from build123d import *

# Parameters (mm, degrees)
SKETCH_1_R          = 235
EXTRUDE_1_DEPTH     = 5
SKETCH_2_R          = 235
SKETCH_2_R_2        = 230
EXTRUDE_2_DEPTH     = 170
CUT_EXTRUDE_1_DEPTH = 376.599520766
EXTRUDE_START       = -5
EXTRUDE_3_DEPTH     = 5
EXTRUDE_4_DEPTH     = 5
SKETCH_6_R          = 2
CUT_EXTRUDE_2_DEPTH = 5
FILLET_1_R          = 3
EXTRUDE_5_DEPTH     = 5
FILLET_2_R          = 10
FILLET_3_R          = 10
SKETCH_8_R          = 2
CUT_EXTRUDE_3_DEPTH = 5
FILLET_4_R          = 10
EXTRUDE_6_DEPTH     = 4
FILLET_5_R          = 3
EXTRUDE_7_DEPTH     = 20
CUT_EXTRUDE_START   = 120
SKETCH_12_W         = 22.896395415
SKETCH_12_H         = 51.404652451
CUT_EXTRUDE_5_DEPTH = 120
SKETCH_13_W         = 30
SKETCH_13_H         = 30
CUT_EXTRUDE_6_DEPTH = 378.955023951
FILLET_6_R          = 5
CUT_EXTRUDE_7_DEPTH = 10
SKETCH_15_R         = 1.5
CUT_EXTRUDE_8_DEPTH = 10
CHAMFER_1_SIZE      = 0.5
SKETCH_16_R         = 2
CUT_EXTRUDE_9_DEPTH = 10
CHAMFER_2_SIZE      = 0.5


with BuildPart() as part:
    # 草图1 → 凸台-拉伸1 (new body)
    with BuildSketch(Plane(origin=(0, 0, 0), x_dir=(0, 0, -1), z_dir=(1, 0, 0))):
        Circle(SKETCH_1_R)
    extrude(amount=EXTRUDE_1_DEPTH)

    # 草图2 → 凸台-拉伸2 (add)
    with BuildSketch(Plane(origin=(5, 0, 0), x_dir=(0, 0, -1), z_dir=(1, 0, 0))):
        Circle(SKETCH_2_R)
        Circle(SKETCH_2_R_2, mode=Mode.SUBTRACT)
    extrude(amount=EXTRUDE_2_DEPTH)

    # 草图3 → 切除-拉伸1 (cut, through all)
    with BuildSketch(Plane.ZY):
        Polygon((0, 0), (0, 250), (330.887429436, 250), (330.887429436, -253.432712339), (-250, -253.432712339), (-250, 0), align=None)
    extrude(amount=-CUT_EXTRUDE_1_DEPTH, mode=Mode.SUBTRACT)

    # 草图4 → 凸台-拉伸3 (add)
    with BuildSketch(Plane(origin=(167, 0, 0), x_dir=(0, 0, -1), z_dir=(1, 0, 0)).offset(EXTRUDE_START)):
        with BuildLine():
            Line((170.570968163, 130.883707237), (182.471268267, 140.015128672))
            ThreePointArc((182.471268267, 140.015128672), (162.634559673, 162.634559673), (140.015128672, 182.471268267))
            Line((140.015128672, 182.471268267), (130.883707237, 170.570968163))
            ThreePointArc((130.883707237, 170.570968163), (152.027957955, 152.027957955), (170.570968163, 130.883707237))
        make_face()
    extrude(amount=EXTRUDE_3_DEPTH)

    # 草图5 → 凸台-拉伸4 (add)
    with BuildSketch(Plane(origin=(59, 0, 0), x_dir=(0, 0, -1), z_dir=(1, 0, 0)).offset(EXTRUDE_START)):
        with BuildLine():
            Line((170.570968163, 130.883707237), (182.471268267, 140.015128672))
            ThreePointArc((182.471268267, 140.015128672), (162.634559673, 162.634559673), (140.015128672, 182.471268267))
            Line((140.015128672, 182.471268267), (130.883707237, 170.570968163))
            ThreePointArc((130.883707237, 170.570968163), (152.027957955, 152.027957955), (170.570968163, 130.883707237))
        make_face()
    extrude(amount=EXTRUDE_4_DEPTH)

    # 草图6 → 切除-拉伸2 (cut)
    with BuildSketch(Plane(origin=(167, 0, 0), x_dir=(0, 0, -1), z_dir=(1, 0, 0))):
        with Locations((146.301163465, 168.30023639)):
            Circle(SKETCH_6_R)
        with Locations((168.30023639, 146.301163465)):
            Circle(SKETCH_6_R)
    extrude(amount=-CUT_EXTRUDE_2_DEPTH, mode=Mode.SUBTRACT)

    # 圆角1
    fillet_1_edges = [part.edges().sort_by_distance(p)[0] for p in [
        (5, 162.634559673, -162.634559673),
        (0, 166.170093579, -166.170093579),
    ]]
    fillet(fillet_1_edges, radius=FILLET_1_R)

    # 草图7 → 凸台-拉伸5 (add)
    with BuildSketch(Plane(origin=(175, 0, 0), x_dir=(0, 0, -1), z_dir=(1, 0, 0))):
        with BuildLine():
            Line((170.570968163, 130.883707237), (186.438034968, 143.058935817))
            ThreePointArc((186.438034968, 143.058935817), (166.170093579, 166.170093579), (143.058935817, 186.438034968))
            Line((143.058935817, 186.438034968), (130.883707237, 170.570968163))
            ThreePointArc((130.883707237, 170.570968163), (152.027957955, 152.027957955), (170.570968163, 130.883707237))
        make_face()
    extrude(amount=EXTRUDE_5_DEPTH)

    # 圆角2
    # the kernel refuses this fillet: 10 mm, written as the material it adds along each edge
    with BuildSketch(Plane(origin=(175, 203.61463864, -156.239007376), x_dir=(0, 0.6087614290087151, 0.7933533402912394), z_dir=(0, -0.7933533402912395, 0.6087614290087151))) as fillet_2_piece_1_section:
        with BuildLine():
            CenterArc((8.660254038, -10), FILLET_2_R, 90, 60)
            Line((0, -5), (0, 0))
            Line((0, 0), (8.660254038, 0))
        make_face()
    fillet_2_piece_1 = extrude(amount=48.301270189, mode=Mode.PRIVATE)
    fillet_2_piece_1 = fillet_2_piece_1 & Plane(origin=(176.322425454, 0, 0), x_dir=(0, 0, -1), z_dir=(-1, 0, 0)) * Cylinder(235, 132, mode=Mode.PRIVATE)
    fillet_2_piece_1 = fillet_2_piece_1 - Plane(origin=(176.322425454, 0, 0), x_dir=(0, 0, -1), z_dir=(-1, 0, 0)) * Cylinder(230, 132, mode=Mode.PRIVATE)
    add(fillet_2_piece_1)
    with BuildSketch(Plane(origin=(175, 126.835057113, -165.294664595), x_dir=(0, -0.7933533402912374, -0.6087614290087175), z_dir=(0, 0.6087614290087178, -0.7933533402912375))) as fillet_2_piece_2_section:
        with BuildLine():
            CenterArc((8.660254038, -10), FILLET_2_R, 90, 60)
            Line((0, -5), (0, 0))
            Line((0, 0), (8.660254038, 0))
        make_face()
    fillet_2_piece_2 = extrude(amount=48.301270189, mode=Mode.PRIVATE)
    fillet_2_piece_2 = fillet_2_piece_2 & Plane(origin=(176.322425454, 0, 0), x_dir=(0, 0, -1), z_dir=(-1, 0, 0)) * Cylinder(235, 132, mode=Mode.PRIVATE)
    fillet_2_piece_2 = fillet_2_piece_2 - Plane(origin=(176.322425454, 0, 0), x_dir=(0, 0, -1), z_dir=(-1, 0, 0)) * Cylinder(230, 132, mode=Mode.PRIVATE)
    add(fillet_2_piece_2)

    # 圆角3
    fillet_3_edges = [part.edges().sort_by_distance(p)[0] for p in [
        (164.5, 130.883707237, -170.570968163),
        (164.5, 170.570968163, -130.883707237),
        (177.5, 170.570968163, -130.883707237),
        (177.5, 130.883707237, -170.570968163),
    ]]
    fillet(fillet_3_edges, radius=FILLET_3_R)

    # 草图8 → 切除-拉伸3 (cut)
    with BuildSketch(Plane(origin=(180, 0, 0), x_dir=(0, 0, -1), z_dir=(1, 0, 0))):
        with Locations((168.30023639, 146.301163465)):
            Circle(SKETCH_8_R)
        with Locations((146.301163465, 168.30023639)):
            Circle(SKETCH_8_R)
    extrude(amount=-CUT_EXTRUDE_3_DEPTH, mode=Mode.SUBTRACT)

    # 圆角4
    fillet_4_edges = [part.edges().sort_by_distance(p)[0] for p in [
        (56.5, 130.883707237, -170.570968163),
        (56.5, 170.570968163, -130.883707237),
    ]]
    fillet(fillet_4_edges, radius=FILLET_4_R)

    # 草图10 → 凸台-拉伸6 (add)
    with BuildSketch(Plane.XZ):
        with BuildLine():
            Line((0, -154), (0, -232))
            ThreePointArc((0, -232), (0.878679656, -234.121320344), (3, -235))
            Line((3, -235), (175, -235))
            Line((175, -235), (175, -154))
            Line((175, -154), (0, -154))
        make_face()
    extrude(amount=EXTRUDE_6_DEPTH)

    # 圆角5
    fillet_5_edges = [part.edges().sort_by_distance(p)[0] for p in [
        (0.878679656, -4, -234.121320344),
        (89, -4, -235),
        (0, -4, -193),
    ]]
    fillet(fillet_5_edges, radius=FILLET_5_R)

    # 草图11 → 凸台-拉伸7 (add)
    with BuildSketch(Plane.ZY):
        with BuildLine():
            Line((0, 224), (0, 221))
            ThreePointArc((0, 221), (-24.121230247, 215.937839886), (-44.172276172, 201.605541713))
            Line((-44.172276172, 201.605541713), (-46.2953836, 203.72864914))
            ThreePointArc((-46.2953836, 203.72864914), (-25.269498453, 218.710072326), (0, 224))
        make_face()
        with BuildLine():
            Line((0, 98), (0, 101))
            ThreePointArc((0, 101), (-24.121230247, 106.062160114), (-44.172276172, 120.394458287))
            Line((-44.172276172, 120.394458287), (-46.2953836, 118.27135086))
            ThreePointArc((-46.2953836, 118.27135086), (-25.269498453, 103.289927674), (0, 98))
        make_face()
        with BuildLine():
            Line((-50.754310162, 129), (-53.214501999, 127.27735513))
            ThreePointArc((-53.214501999, 127.27735513), (-63, 161), (-53.214501999, 194.72264487))
            Line((-53.214501999, 194.72264487), (-50.754310162, 193))
            ThreePointArc((-50.754310162, 193), (-60, 161), (-50.754310162, 129))
        make_face()
    extrude(amount=EXTRUDE_7_DEPTH)

    # 草图12 → 切除-拉伸5 (cut)
    with BuildSketch(Plane(origin=(0, 0, 0), x_dir=(1, 0, 0), z_dir=(0, 1, 0)).offset(CUT_EXTRUDE_START)):
        with Locations((-13.448197708, 2.297673774)):
            Rectangle(SKETCH_12_W, SKETCH_12_H)
    extrude(amount=CUT_EXTRUDE_5_DEPTH, mode=Mode.SUBTRACT)

    # 草图13 → 切除-拉伸6 (cut, through all)
    with BuildSketch(Plane(origin=(0, 0, 0), x_dir=(1, 0, 0), z_dir=(0, 1, 0))):
        with Locations((85, 0)):
            Rectangle(SKETCH_13_W, SKETCH_13_H)
    extrude(amount=CUT_EXTRUDE_6_DEPTH, mode=Mode.SUBTRACT)

    # 圆角6
    fillet_6_edges = [part.edges().sort_by_distance(p)[0] for p in [
        (70, 232.015568171, -15),
        (100, 232.015568171, -15),
    ]]
    fillet(fillet_6_edges, radius=FILLET_6_R)

    # 草图14 → 切除-拉伸7 (cut)
    with BuildSketch(Plane.ZY):
        with BuildLine():
            Line((-82.5, 10.5), (-82.5, 0))
            Line((-82.5, 0), (-112.5, 0))
            Line((-112.5, 0), (-112.5, 10.5))
            ThreePointArc((-112.5, 10.5), (-97.5, 25.5), (-82.5, 10.5))
        make_face()
    extrude(amount=-CUT_EXTRUDE_7_DEPTH, mode=Mode.SUBTRACT)

    # 草图15 → 切除-拉伸8 (cut)
    with BuildSketch(Plane.ZY):
        with Locations((-21, 21)):
            Circle(SKETCH_15_R)
    extrude(amount=-CUT_EXTRUDE_8_DEPTH, mode=Mode.SUBTRACT)

    # 倒角1
    chamfer_1_edges = [part.edges().sort_by_distance(p)[0] for p in [
        (0, 21, -22.5),
    ]]
    chamfer(chamfer_1_edges, length=CHAMFER_1_SIZE)

    # 草图16 → 切除-拉伸9 (cut)
    with BuildSketch(Plane.ZY):
        with Locations((-159.099025767, 137.885822331)):
            Circle(SKETCH_16_R)
        with Locations((-137.885822331, 159.099025767)):
            Circle(SKETCH_16_R)
    extrude(amount=-CUT_EXTRUDE_9_DEPTH, mode=Mode.SUBTRACT)

    # 倒角2
    chamfer_2_edges = [part.edges().sort_by_distance(p)[0] for p in [
        (0, 137.885822331, -161.099025767),
        (0, 159.099025767, -139.885822331),
    ]]
    chamfer(chamfer_2_edges, length=CHAMFER_2_SIZE)


solid = part.part
Read the model definition and answer for the solid it produces. Units are mm, in the model's axes. A direction names the side the tool comes from. Coordinates: 2 decimals unless noted, no trailing zeros. Write each loop counter-clockwise with the first axis right and the second up, starting at its lowest first coordinate (ties: lowest second). Pieces come first, ordered by that corner, then holes. Notation, with made-up numbers: M 11,22 L 52,22 A20 ccw 52,31 Z; hole C 64,-7 d5. An arc over 180 degrees is marked long. Use a Markdown table: item, result.
Q1. Which of the six approach directions +Z, -Z, +X, -X, +Y, -Y give full straight-line access (tool end or side, diameter ignored) to faces 4 (the face through (-9.86, 103.437, -25.603)), 5 (the face through (-10, 161, -60)), 6 (the face through (-9.86, 212.93, -35.67))?
Answer block:
| item | result |
|---|---|
| face 4 | -Z, -X, -Y |
| face 5 | +Z, -X |
| face 6 | -Z, -X, +Y |
Q2. Straight lines are drawn through the part: L1, parallel to X at y = 9.5, z = -124.5; L2, parallel to Y at x = -6, z = -38.5; L3, parallel to Y at x = 2.15, z = -21. For each, find the intervals that lie inside material, in ascending order. Write a range as [from, to].
Answer block:
| item | result |
|---|---|
| L1 | x = [0, 5] |
| L2 | y = [111.13, 114.98], [207.02, 210.87] |
| L3 | y = [0, 19.5], [22.5, 233.94] |
Q3. The part is cut by section B-B, the plane x = 13.5. Write down the section's boundary in (y, z).
Answer block:
| item | result |
|---|---|
| outline | M -4,-232 A3 ccw -1,-235 L 0,-235 A235 ccw 235,0 L 230,0 A230 cw 0,-230 L 0,-154 L -4,-154 Z |
Q4. The part is cut by section A-A, the plane x = 80. Write down the section's boundary in (y, z), then the cut area to 3 significant figures.
Answer block:
| item | result |
|---|---|
| outline | M -4,-232 A3 ccw -1,-235 L 0,-235 A235 ccw 234.52,-15 L 229.51,-15 A230 cw 0,-230 L 0,-154 L -4,-154 Z |
| area | 2,070 mm2 |
Q5. Determine the mould class of faces 1 (the face through (162, 159, -158)), 2 (the face through (175, 220, -68)), 3 (the face through (88, -4, -192)) for opening direction Y: released by +Y, released by -Y, zero draft, split by the parting line, or undercut.
Answer block:
| item | result |
|---|---|
| face 1 | undercut |
| face 2 | zero draft |
| face 3 | released by -Y |
Q6. Each of these flat-tipped pins is pushed along its axis until it touches: pin 1 Ø6.5 at (y, z) = (168.3, -146.3) entering from -X; pin 2 Ø3 at (y, z) = (112.5, -98) entering from +X; pin 3 Ø4 at (x, z) = (111.5, -38.5) entering from +Y. Where does it stop, or does it pass through?
Answer block:
| item | result |
|---|---|
| pin 1 | stops at x = 0 |
| pin 2 | stops at x = 5 |
| pin 3 | stops at y = 232.15 |
